Design review of the part shown in the three views and the two pictorial views. Dimensions are in mm from the part's minimum x, y and z. A direction names the side the tool comes from. Give positions to 0.01 mm unless a question says otherwise; leave off trailing zeros. Order: outer loops, then holes, each group sorted by start corner. A loop starts at its lowest first (then second) coordinate and runs counter-clockwise, first axis right, second up. Notation, with made-up numbers: (-10.75, 55.5) - (23.25, 55.5) arc R30 ccw to (23.25, 88.5) - close; hole circle Ø6 at (58, 6.5). An arc over 180 degrees is marked (long way). Put each result on its own line as item: value.
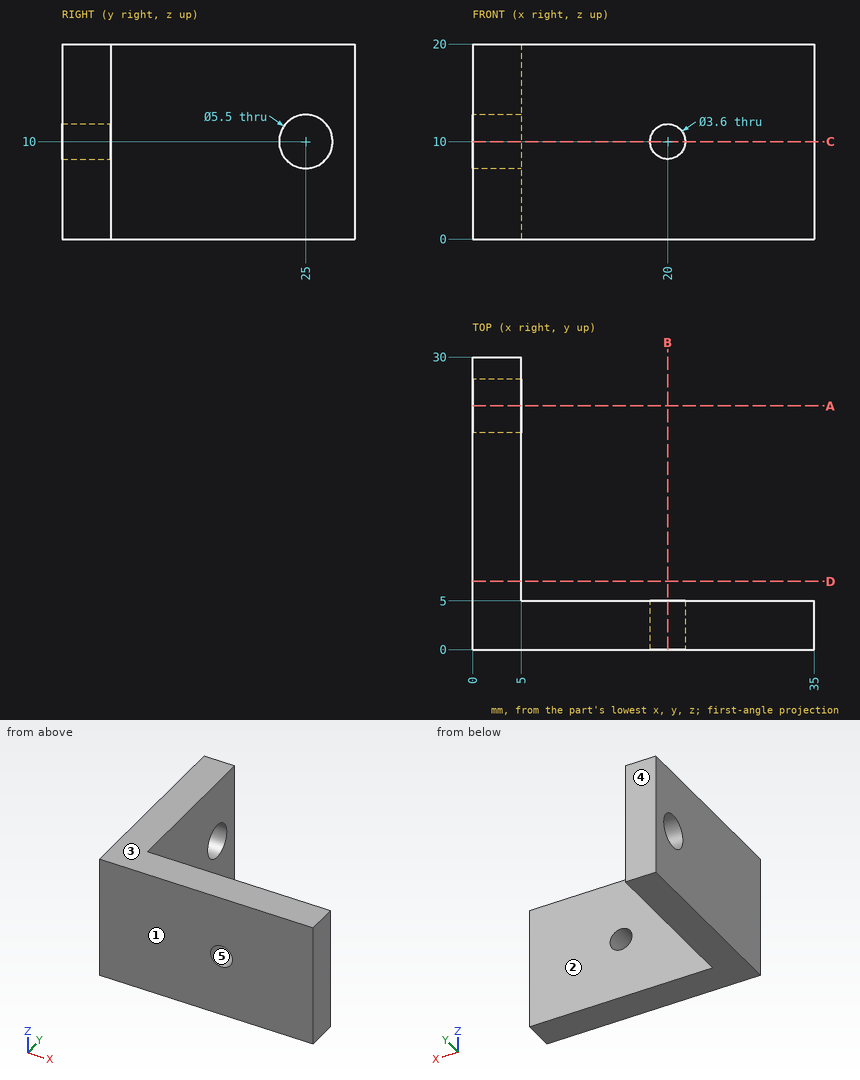
(1) Take a section at D-D, the plane y = 7. Write out the cut boundary in (x, z).
The answers:
outline: (0, 0) - (5, 0) - (5, 20) - (0, 20) - close
(2) Take a section at C-C, the plane z = 10. Write out the cut boundary in (x, y).
The answers:
outline: (0, 0) - (18.2, 0) - (18.2, 5) - (5, 5) - (5, 22.25) - (0, 22.25) - close; (0, 27.75) - (5, 27.75) - (5, 30) - (0, 30) - close; (21.8, 0) - (35, 0) - (35, 5) - (21.8, 5) - close
(3) Clearance check with flat-ended pins moving along their axes: pin 1 Ø10 at (x, z) = (19, 12.5) entering from +Y; pin 2 Ø4.5 at (y, z) = (25, 10) entering from +X; pin 3 Ø6 at (y, z) = (21.5, 13) entering from +X. State where each tip first meets the part, or that it passes through.
The answers:
pin 1: y = 5
pin 2: through
pin 3: x = 5
(4) Wall thickness on L1, parallel to X at y = 3.8, z = 10; L2, parallel to Z at x = 20, y = 1.55; L3, parallel to Y at x = 2.7, z = 10: over which ranges is each line inside the solid? List them lowest first.
The answers:
L1: 0 to 18.2, 21.8 to 35
L2: 0 to 8.2, 11.8 to 20
L3: 0 to 22.25, 27.75 to 30
(5) Take a section at B-B, the plane x = 20. Write out the cut boundary in (y, z), then the cut area to 3 significant figures.
The answers:
outline: (0, 0) - (5, 0) - (5, 8.2) - (0, 8.2) - close; (0, 11.8) - (5, 11.8) - (5, 20) - (0, 20) - close
area: 82.0 mm^2
(6) For the marked faces 1 and 2, list the 3-axis set-ups (+Z, -Z, +X, -X, +Y, -Y) from which the entire face can be reached by the end or side of a thin tool; tool diameter is ignored.
The answers:
face 1: +Z, -Z, +X, -X, -Y
face 2: +Z, -Z, +X, +Y
(7) Take a section at A-A, the plane y = 25. Write out the cut boundary in (x, z), then the cut area to 3 significant figures.
The answers:
outline: (0, 0) - (5, 0) - (5, 7.25) - (0, 7.25) - close; (0, 12.75) - (5, 12.75) - (5, 20) - (0, 20) - close
area: 72.5 mm^2
(8) The part is to be moulded in two halves that separate along Z. For the marked faces 3, 4 and 5, say which applies: pulls with the +Z half, pulls with the -Z half, needs draft (parallel to the pull), parting line crosses it, or undercut.
The answers:
face 3: pulls with the +Z half
face 4: needs draft
face 5: undercut
